```python
from build123d import *

# Parameters (mm, degrees)
BOSS_EXTRUDE1_DEPTH = 6
SKETCH4_R           = 6
BOSS_EXTRUDE2_DEPTH = 6
SKETCH3_R           = 6
SKETCH3_R_2         = 2
CUT_EXTRUDE1_DEPTH  = 383.864205692


with BuildPart() as part:
    # Sketch2 → Boss-Extrude1 (new body)
    with BuildSketch(Plane(origin=(0, 0, 0), x_dir=(0, 0, -1), z_dir=(1, 0, 0))):
        Polygon((6, 382), (-25, 351), (-25, 25), (6, -6), align=None)
    extrude(amount=BOSS_EXTRUDE1_DEPTH)

    # Sketch4 → Boss-Extrude2 (add)
    with BuildSketch(Plane.ZY):
        with Locations((12, 12)):
            Circle(SKETCH4_R)
    extrude(amount=-BOSS_EXTRUDE2_DEPTH)

    # Sketch3 → Cut-Extrude1 (cut, through all)
    with BuildSketch(Plane(origin=(0, 0, 0), x_dir=(0, 0, -1), z_dir=(1, 0, 0))):
        with Locations((-12, 364)):
            Circle(SKETCH3_R)
        with Locations((-12, 12)):
            Circle(SKETCH3_R_2)
    extrude(amount=CUT_EXTRUDE1_DEPTH, mode=Mode.SUBTRACT)


solid = part.part
```
Design review of the part built by this model. Coordinates are the model's own, in mm. A direction names the side the tool comes from. Coordinates: 2 decimals unless noted, no trailing zeros. Order: outer loops, then holes, each group sorted by start corner. A loop starts at its lowest first (then second) coordinate and runs counter-clockwise, first axis right, second up.
1) Take a section at A-A, the plane x = 4.45. Give the boundary of the cut face in (y, z).
2) Mouldability with a two-part tool opening along Y and no side actions: class faces 1 (the cylindrical face through (2.958, 359.665, 7.852)), 2 (the flat face through (3, 190, 25)), 3 (the flat face through (3, 1, 1)) as +Y half, -Y half, draft (parallel to the pull), parting line (faces both ways), or undercut.
3) Take a section at B-B, the plane y = 364. Give the boundary of the cut face in (x, z), and give its area (3 significant figures).
4) Clearance check with a flat-ended pin moving along its axis: pin 1 (3 mm diameter, centred on y = 12, z = 12, fed in from +X). State where the tip first meets the part, or that it passes through.
5) Wall thickness on line 1 along Y through (x, z) = (4.3, 12); line 2 along Z through (x, y) = (2.6, 12); line 3 along Z through (x, y) = (2, 18): over which ranges is each line inside the solid? List them lowest first.
6) For faces 4 (the flat face through (3, 375, 1)), 5 (the flat face through (3, 21, 21)), list the 3-axis set-ups (+Z, -Z, +X, -X, +Y, -Y) from which the entire face can be reached by the end or side of a thin tool; tool diameter is ignored.
Returned:
1. outline: (-6, -6) - (382, -6) - (368.24, 7.76) arc R6 cw to (359.76, 16.24) - (351, 25) - (25, 25) - (16.24, 16.24) arc R6 ccw to (7.76, 7.76) - close; hole circle Ø4 at (12, 12)
2. face 1: undercut
2. face 2: draft
2. face 3: -Y half
3. outline: (0, -6) - (6, -6) - (6, 6) - (0, 6) - close
3. area: 72.0 mm2
4. pin 1: passes through
5. line 1: y = 6 to 10, 14 to 358
5. line 2: z = -6 to 10, 14 to 18
5. line 3: z = -6 to 18
6. face 4: +Z, +X, -X, +Y
6. face 5: +Z, +X, -X
